from build123d import *

# Parameters (mm, degrees)
F0_R     = 1.23227
F0_R_2   = 1.246014
F1_DEPTH = 2.9718


with BuildPart() as f1:
    # F0 (on Top) → F1 (new body)
    with BuildSketch(Plane.XY):
        Polygon((-50.820782, -76.199999), (50.822706, -76.199999), (50.822706, -10.159999), (47.848982, -10.159999), (47.848982, -4.600307), (47.848982, -1.456227), (42.741386, -1.456227), (42.741967, -3.213268), (40.278167, -3.213268), (40.278167, -1.4605), (35.149562, -1.4605), (35.149562, 0), (35.149562, 1.4605), (40.278167, 1.4605), (40.278167, 3.136732), (42.818167, 3.136732), (42.818167, 1.4605), (47.848982, 1.456228), (47.848982, 10.160001), (50.82015, 10.160001), (50.82015, 35.559999), (47.848982, 35.559999), (47.848982, 44.263772), (42.817586, 44.263772), (42.817586, 42.58754), (40.277586, 42.58754), (40.277586, 44.263772), (35.148982, 44.263772), (35.149562, 47.176227), (40.277586, 47.176227), (40.277586, 48.928995), (42.741386, 48.928995), (42.741386, 47.176227), (47.848982, 47.176227), (47.848982, 55.879999), (50.820782, 55.879999), (50.820782, 76.199999), (35.580782, 76.199999), (35.580782, 73.232112), (26.879027, 73.241051), (26.879027, 68.122951), (28.561365, 68.122951), (28.561365, 65.582951), (26.844848, 65.582951), (26.844848, 60.532112), (25.384348, 60.532112), (23.923848, 60.532112), (23.923848, 65.641274), (22.209348, 65.641274), (22.209348, 68.105074), (23.923848, 68.105074), (23.923848, 73.232112), (15.218057, 73.232112), (15.218057, 76.232044), (-0.021943, 76.232044), (-15.261943, 76.232044), (-15.261943, 73.232112), (-23.967733, 73.232112), (-23.967733, 68.122951), (-22.24267, 68.122951), (-22.24267, 65.582951), (-23.95717, 65.582951), (-23.95717, 60.560244), (-25.41767, 60.560244), (-26.87817, 60.560244), (-26.87817, 65.659151), (-28.594688, 65.659151), (-28.594688, 68.122951), (-26.880188, 68.122951), (-26.880188, 73.241051), (-35.581943, 73.232112), (-35.582706, 76.203912), (-50.822706, 76.199999), (-50.822706, 55.879999), (-47.850906, 55.879999), (-47.850906, 47.209491), (-42.726061, 47.209491), (-42.726061, 48.940623), (-40.186061, 48.940623), (-40.186061, 47.209491), (-35.150906, 47.209491), (-35.150906, 45.757536), (-35.150906, 44.297036), (-40.262261, 44.297036), (-40.262261, 42.565904), (-42.726061, 42.565904), (-42.726061, 44.297036), (-47.850906, 44.297036), (-47.850906, 35.559999), (-50.822706, 35.559999), (-50.822706, 10.159999), (-47.850906, 10.159999), (-47.815394, 1.427236), (-42.724717, 1.427236), (-42.724717, 3.158368), (-40.260917, 3.158368), (-40.260917, 1.427236), (-35.149562, 1.427236), (-35.149562, -0.033264), (-35.149562, -1.493764), (-40.260917, -1.493764), (-40.260917, -3.224896), (-42.724717, -3.224896), (-42.724717, -1.493764), (-47.815546, -1.493764), (-47.850906, -10.159999), (-50.820782, -10.159999), align=None)
        with Locations((-49.082806, 22.89018)):
            Circle(F0_R, mode=Mode.SUBTRACT)
        with Locations((-0.010971, 74.478078)):
            Circle(F0_R_2, mode=Mode.SUBTRACT)
        with Locations((49.082806, 22.89018)):
            Circle(F0_R, mode=Mode.SUBTRACT)
    extrude(amount=F1_DEPTH)


solid = f1.part
For this review, take the finished solid that the model builds, in its own axes (mm). A direction names the side the tool comes from. Give positions to 0.01 mm unless a question says otherwise; leave off trailing zeros. Order: outer loops, then holes, each group sorted by start corner. A loop starts at its lowest first (then second) coordinate and runs counter-clockwise, first axis right, second up. Notation, with made-up numbers: (-7.75, -22.5) -> (14.25, -22.5) arc R14 ccw to (14.25, -14.5) -> close; hole circle Ø6 at (8.25, -34). An arc over 180 degrees is marked (long way). Write item = value, one per line.
1) Draft analysis for pull direction Y (two halves, no side actions). For faces 6 (the face through (-1, -76.2, 1)), 7 (the face through (-49, 35.56, 1)), 8 (the face through (-20, 73.232, 1)), state which applies: pulls with the +Y half, pulls with the -Y half, needs draft (parallel to the pull), parting line crosses it, or undercut.
Findings:
face_6 = pulls with the -Y half
face_7 = undercut
face_8 = pulls with the +Y half
2) We need section C-C, the plane x = -38.5. Give the boundary of the cut face in (y, z), and give its area (3 significant figures).
Findings:
outline = (-76.2, 0) -> (-1.49, 0) -> (-1.49, 2.97) -> (-76.2, 2.97) -> close; (1.43, 0) -> (44.3, 0) -> (44.3, 2.97) -> (1.43, 2.97) -> close; (47.21, 0) -> (76.2, 0) -> (76.2, 2.97) -> (47.21, 2.97) -> close
area = 436 mm^2
3) We need section B-B, the plane y = 50.5. Give the boundary of the cut face in (x, z), and give its area (3 significant figures).
Findings:
outline = (-47.85, 0) -> (47.85, 0) -> (47.85, 2.97) -> (-47.85, 2.97) -> close
area = 284 mm^2
4) To check wall thickness, follow L1, parallel to Y at x = -38, z = 1.5; L2, parallel to X at y = 48, z = 2.3; L3, parallel to X at y = 69.5, z = 1.35. State the ranges of each line that lie inside material, in increasing order. Write a range as from..to.
Findings:
L1 = -76.2..-1.49, 1.43..44.3, 47.21..76.2
L2 = -47.85..-42.73, -40.19..40.28, 42.74..47.85
L3 = -50.82..-26.88, -23.97..23.92, 26.88..50.82
5) For faces 1 (the face through (38, 47.176, 1)), 2 (the face through (-50.821, -43, 1)), 3 (the face through (50.821, 66, 1)), 4 (the face through (-38, 44.297, 1)), 5 (the face through (-26.878, 63, 1)), list the 3-axis set-ups (+Z, -Z, +X, -X, +Y, -Y) from which the entire face can be reached by the end or side of a thin tool; tool diameter is ignored.
Findings:
face_1 = +Z, -Z, +X
face_2 = +Z, -Z, -X, +Y, -Y
face_3 = +Z, -Z, +X, +Y, -Y
face_4 = +Z, -Z, -X
face_5 = +Z, -Z, +Y
6) Insertion check: pin 1 (0.5 mm diameter, centred on y = 2.5, z = 1, fed in from +X); pin 2 (1.5 mm diameter, centred on x = 13.5, y = -50, fed in from -Z); pin 3 (1.5 mm diameter, centred on y = 46, z = 1, fed in from +X); pin 4 (1.5 mm diameter, centred on y = 0, z = 1.5, fed in from -X). Each pin has a flat end and moves straight along its axis. Give the tip position at first contact, or say it passes through.
Findings:
pin_1 = 47.85
pin_2 = 0
pin_3 = 35.15
pin_4 = -35.15
7) We need section D-D, the plane z = 2.05. Count the separate pieces of the cut face and the enclosed holes in it, and give its area (3 significant figures).
Findings:
separate_pieces = 1
enclosed_holes = 3
area = 14,800 mm^2
8) We need section A-A, the plane x = 38. Give the boundary of the cut face in (y, z), and give its area (3 significant figures).
Findings:
outline = (-76.2, 0) -> (-1.46, 0) -> (-1.46, 2.97) -> (-76.2, 2.97) -> close; (1.46, 0) -> (44.26, 0) -> (44.26, 2.97) -> (1.46, 2.97) -> close; (47.18, 0) -> (76.2, 0) -> (76.2, 2.97) -> (47.18, 2.97) -> close
area = 436 mm^2
